Model file for the job. Use its own axes, mm. Face numbers are marked on the shaded views. A direction names the side the tool comes from. Coordinates: 2 decimals unless noted, no trailing zeros. Order: outer loops, then holes, each group sorted by start corner. A loop starts at its lowest first (then second) coordinate and runs counter-clockwise, first axis right, second up. Notation, with made-up numbers: (31, 22.5) - (37, 22.5) arc R16 ccw to (37, 31.5) - close; hole circle Ø10 at (24, -35.5). An arc over 180 degrees is marked (long way). Put each result on its own line as item: value. Start each with the question number.
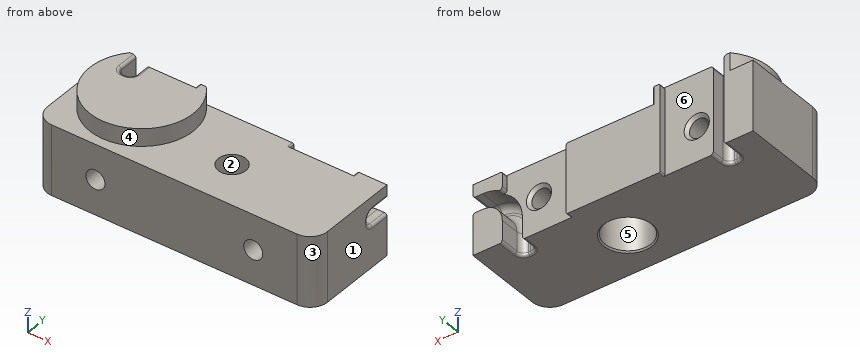
```python
from build123d import *

# Parameters (mm, degrees)
SKETCH1_W                       = 50.8
SKETCH1_H                       = 17.4752
BOSS_EXTRUDE1_DEPTH             = 12.7
BOSS_EXTRUDE2_DEPTH             = 3.175
SKETCH12_W                      = 11.5824
SKETCH12_H                      = 31.04642485
SKETCH12_H_2                    = 37.220312072
CUT_EXTRUDE5_DEPTH              = 1.143
F_9_0_196_DIAMETER_HOLE1_D      = 4.9784
FILLET1_R                       = 3.175
F_8_32_TAPPED_HOLE2_D           = 3.4544
F_8_32_TAPPED_HOLE2_CSINK_D     = 4.572
F_8_32_TAPPED_HOLE2_CSINK_ANGLE = 90
SKETCH11_W                      = 2.794
SKETCH11_H                      = 23.198016048
CUT_EXTRUDE4_DEPTH              = 4.699
FILLET2_R                       = 1.1938
FILLET3_R                       = 0.508
FILLET4_R                       = 0.254
SKETCH16_R                      = 4.1656
CUT_EXTRUDE6_DEPTH              = 6.35
CHAMFER1_SIZE                   = 0.254
FILLET8_R                       = 0.508


with BuildPart() as part:
    # Sketch1 → Boss-Extrude1 (new body)
    with BuildSketch(Plane.XY):
        with Locations((0, -8.7376)):
            Rectangle(SKETCH1_W, SKETCH1_H)
    extrude(amount=-BOSS_EXTRUDE1_DEPTH)

    # Sketch2 → Boss-Extrude2 (add)
    with BuildSketch(Plane.XY):
        with BuildLine():
            Line((-21.228396302, 0), (-7.372003698, 0))
            ThreePointArc((-7.372003698, 0), (-14.3002, -15.748), (-21.228396302, 0))
        make_face()
    extrude(amount=BOSS_EXTRUDE2_DEPTH)

    # Sketch12 → Cut-Extrude5 (cut)
    with BuildSketch(Plane(origin=(0, 0, 0), x_dir=(1, 0, 0), z_dir=(0, 1, 0))):
        with Locations((14.3002, 4.674371042)):
            Rectangle(SKETCH12_W, SKETCH12_H)
        with Locations((-14.3002, 2.29159367)):
            Rectangle(SKETCH12_W, SKETCH12_H_2)
    extrude(amount=-CUT_EXTRUDE5_DEPTH, mode=Mode.SUBTRACT)

    # #9 (0.196) Diameter Hole1 (through all)
    with Locations(Plane(origin=(33.7312, -2.208443868, 0), x_dir=(1, 0, 0), z_dir=(0, 0, 1))):
        with Locations((-29.247846689, -7.316556132)):
            Hole(F_9_0_196_DIAMETER_HOLE1_D / 2)

    # Fillet1
    fillet1_edges = [part.edges().sort_by_distance(p)[0] for p in [
        (25.4, -17.4752, -6.35),
        (-25.4, -17.4752, -6.35),
    ]]
    fillet(fillet1_edges, radius=FILLET1_R)

    # #8-32 Tapped Hole2 (through all)
    with Locations(Plane(origin=(26.700019519, -1.143, -0.758269739), x_dir=(-1, 0, 0), z_dir=(0, 1, 0))):
        with Locations((12.399819519, -5.591730261), (41.000219519, -5.591730261)):
            CounterSinkHole(F_8_32_TAPPED_HOLE2_D / 2, F_8_32_TAPPED_HOLE2_CSINK_D / 2, counter_sink_angle=F_8_32_TAPPED_HOLE2_CSINK_ANGLE)

    # Sketch11 → Cut-Extrude4 (cut)
    with BuildSketch(Plane(origin=(0, 0, 0), x_dir=(1, 0, 0), z_dir=(0, 1, 0))):
        with BuildLine():
            Line((20.0914, 20.298121943), (20.0914, 8.7376))
            ThreePointArc((20.0914, 8.7376), (21.132928286, 6.223128286), (23.6474, 5.1816))
            Line((23.6474, 5.1816), (32.110940615, 5.1816))
            Line((32.110940615, 5.1816), (32.110940615, 2.3876))
            Line((32.110940615, 2.3876), (23.6474, 2.3876))
            ThreePointArc((23.6474, 2.3876), (19.157271939, 4.247471939), (17.2974, 8.7376))
            Line((17.2974, 8.7376), (17.2974, 20.298121943))
            Line((17.2974, 20.298121943), (20.0914, 20.298121943))
        make_face()
        with Locations((-18.6944, 5.241099364)):
            Rectangle(SKETCH11_W, SKETCH11_H)
    extrude(amount=-CUT_EXTRUDE4_DEPTH, mode=Mode.SUBTRACT)

    # Fillet2
    fillet2_edges = [part.edges().sort_by_distance(p)[0] for p in [
        (24.5237, -4.699, -5.1816),
        (24.5237, -4.699, -2.3876),
        (19.157271939, -4.699, -4.247471939),
        (17.2974, -4.699, -10.7188),
        (20.0914, -4.699, -10.7188),
        (21.132928286, -4.699, -6.223128286),
        (-17.2974, -4.699, -4.7625),
        (-20.0914, -4.699, -4.7625),
    ]]
    fillet(fillet2_edges, radius=FILLET2_R)

    # Fillet3
    fillet3_edges = [part.edges().sort_by_distance(p)[0] for p in [
        (20.0914, -0.5715, -3.476671945),
    ]]
    fillet(fillet3_edges, radius=FILLET3_R)

    # Fillet4
    fillet4_edges = [part.edges().sort_by_distance(p)[0] for p in [
        (-8.509, -0.5715, 3.175),
        (-8.509, -0.5715, -12.7),
        (8.509, -0.5715, -12.7),
        (8.509, -0.5715, 0),
        (20.0914, -0.5715, 0),
    ]]
    fillet(fillet4_edges, radius=FILLET4_R)

    # Sketch16 → Cut-Extrude6 (cut)
    with BuildSketch(Plane(origin=(0, 0, -12.7), x_dir=(-1, 0, 0), z_dir=(0, 0, -1))):
        with Locations((-4.483353311, -9.525)):
            Circle(SKETCH16_R)
    extrude(amount=-CUT_EXTRUDE6_DEPTH, mode=Mode.SUBTRACT)

    # Chamfer1
    chamfer1_edges = [part.edges().sort_by_distance(p)[0] for p in [
        (8.648953311, -9.525, -12.7),
        (6.972553311, -9.525, -6.35),
    ]]
    chamfer(chamfer1_edges, length=CHAMFER1_SIZE)

    # Fillet8
    fillet8_edges = [part.edges().sort_by_distance(p)[0] for p in [
        (25.4, -1.7526, -2.3876),
        (17.2974, -2.3241, -12.7),
        (18.6944, -4.699, -12.7),
        (25.4, -4.699, -3.7846),
        (25.4, -1.7526, -5.1816),
        (-18.6944, -4.699, -12.7),
        (-18.6944, -4.699, 3.175),
        (-17.2974, -2.3241, 3.175),
        (-17.2974, -2.3241, -12.7),
        (20.0914, -1.7526, -12.7),
        (25.4, -4.349344075, -2.737255925),
        (25.4, -4.349344075, -4.831944075),
        (-19.741744075, -4.349344075, -12.7),
        (-19.741744075, -4.349344075, 3.175),
        (-17.647055925, -4.349344075, 3.175),
        (-17.647055925, -4.349344075, -12.7),
        (17.647055925, -4.349344075, -12.7),
        (19.741744075, -4.349344075, -12.7),
        (-20.0914, -1.7526, 3.175),
        (-20.0914, -1.7526, -12.7),
    ]]
    fillet(fillet8_edges, radius=FILLET8_R)


solid = part.part
```
Item 1: Wall check: line 1 along X through (y, z) = (-1.75, -9.5); line 2 along X through (y, z) = (-11.25, -6.75) (3 decimals); line 3 along Z through (x, y) = (0, -15.5). Give the ranges that are in metal, low to high.
Item 2: 3-axis set-ups, long thin cutter, end or side, ignore diameter. For the marked faces 4, 5 and 6: which of +Z, -Z, +X, -X, +Y, -Y reach the whole face in a straight line?
Item 3: Flat gauge pins, fed straight in: pin 1 Ø4.5 at (x, y) = (4.48, -9.52) entering from +Z; pin 2 Ø2.5 at (x, y) = (6.5, -7.5) entering from -Z; pin 3 Ø9.5 at (x, y) = (4.48, -9.52) entering from +Z. Where does each tip first touch, or does it go through?
Item 4: Pull direction Y, two halves, no side cores. Call the marked faces 1, 2 and 3: pulls with the +Y half, pulls with the -Y half, needs draft (parallel to the pull), parting line crosses it, or undercut.
Item 5: Slice it at A-A, the plane y = -7.5. Give the number of separate pieces and of enclosed holes in the cut face, plus the area to 3 significant figures.
Item 6: Slice it at C-C, the plane x = -9. Give the cut face in (y, z) (3 decimals), plus the area to 3 significant figures.
Here are the results:
1. line 1: x = -25.4 to -20.09, -17.3 to 17.3, 20.09 to 25.4
1. line 2: x = -25.4 to -15.98, -12.62 to 0.692, 8.275 to 12.62, 15.98 to 25.4
1. line 3: z = -12.7 to 0
2. face 4: +Z
2. face 5: -Z
2. face 6: +Z, -Z, +Y
3. pin 1: passes through
3. pin 2: stops at z = -6.35
3. pin 3: stops at z = 0
4. face 1: needs draft
4. face 2: undercut
4. face 3: pulls with the -Y half
5. separate pieces: 2
5. enclosed holes: 2
5. area: 621 mm^2
6. outline: (-17.475, -12.7) - (-1.143, -12.7) - (-1.143, 3.175) - (-14.111, 3.175) - (-14.111, 0) - (-17.475, 0) - close
6. area: 249 mm^2
